The drawing under review shows one solid part. Ordinate dimensions are in mm from its lowest x, y, z. Round coordinates to 2 decimals unless told otherwise and drop trailing zeros. Order: outer loops, then holes, each group sorted by start corner. A loop starts at its lowest first (then second) coordinate and runs counter-clockwise, first axis right, second up. Notation, with made-up numbers: (74, 47.5) -> (91, 47.5) arc R21 cw to (91, 66.5) -> close; hole circle Ø9 at (52.5, 83). An arc over 180 degrees is marked (long way). Return JSON: item names as keys, results as strings. Group by question number.
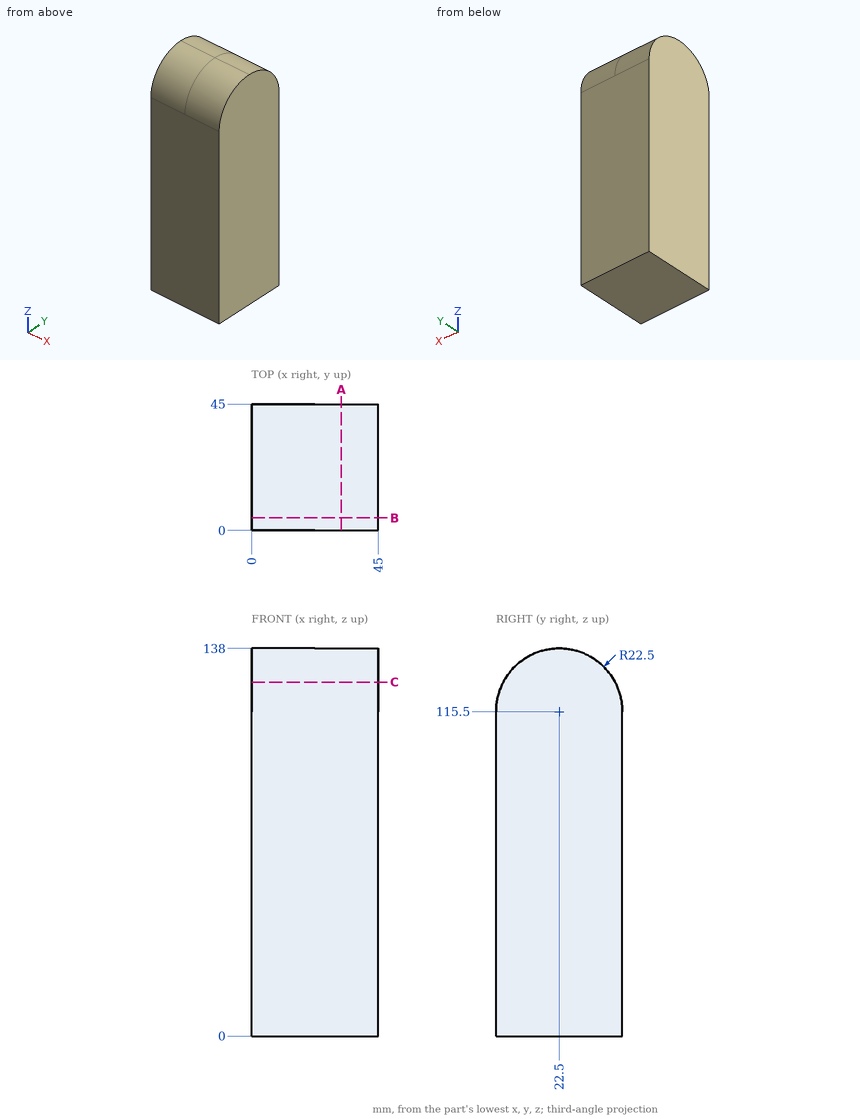
Item 1: Wall thickness on line 1 along Z through (x, y) = (3, 39); line 2 along Z through (x, y) = (39.5, 34); line 3 along Y through (x, z) = (18.5, 120): over which ranges is each line inside the solid? List them lowest first.
Item 2: Insertion check: pin 1 Ø4 at (x, y) = (21.5, 6) entering from +Z; pin 2 Ø1 at (x, y) = (38, 6.5) entering from +Z. Each pin has a flat end and moves straight along its axis. Give the tip position at first contact, or say it passes through.
Item 3: Consider section A-A on x = 32. State the section outline as (y, z) points, plus the area to 3 significant figures.
Item 4: Consider section C-C on z = 126. State the section outline as (x, y) points, plus the area to 3 significant figures.
Item 5: Consider section B-B on y = 4.5. State the section outline as (x, z) points.
Values:
{
 "1": {"line 1": "0 to 130.8", "line 2": "0 to 134.84", "line 3": "0.45 to 44.55"},
 "2": {"pin 1": "z = 132.7", "pin 2": "z = 131.81"},
 "3": {"outline": "(0, 0) -> (45, 0) -> (45, 115.5) arc R22.5 ccw to (0, 115.5) -> close", "area": "5,990 mm^2"},
 "4": {"outline": "(0, 2.6) -> (45, 2.6) -> (45, 42.4) -> (0, 42.4) -> close", "area": "1,790 mm^2"},
 "5": {"outline": "(0, 0) -> (45, 0) -> (45, 129) -> (0, 129) -> close"}
}
